Design review of the part shown in the three views and the two pictorial views. Dimensions are in mm from the part's minimum x, y and z. Give positions to 0.01 mm unless a question says otherwise; leave off trailing zeros. Loops run counter-clockwise (first coordinate to the right, second up) from the corner with the lowest first, then second, coordinate; pieces in that order, holes last.
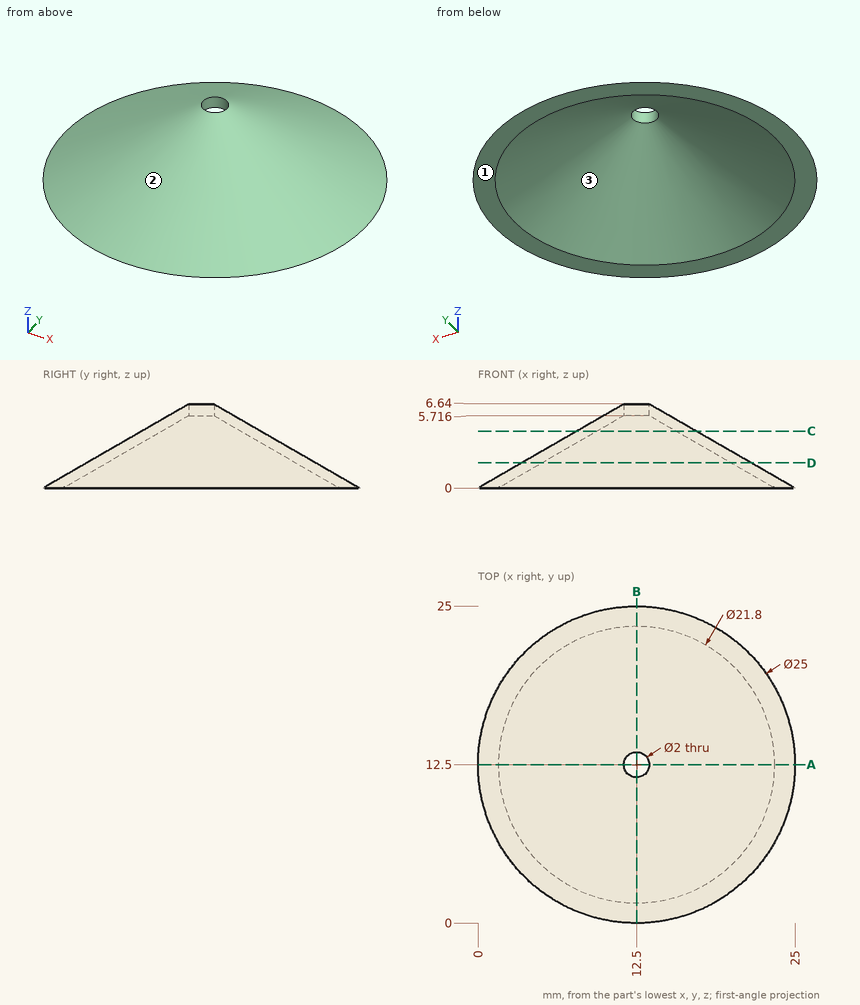
Q1. Insertion check: pin 1 (3 mm diameter, centred on x = 6, y = 15.5, fed in from +Z); pin 2 (1.6 mm diameter, centred on x = 12.5, y = 12.5, fed in from -Z); pin 3 (6 mm diameter, centred on x = 5, y = 19.5, fed in from +Z) (1 decimal); pin 4 (12 mm diameter, centred on x = 20.5, y = 8.5, fed in from +Z). Each pin has a flat end and moves straight along its axis. Give the tip position at first contact, or say it passes through.
Results:
pin 1: stops at z = 3.95
pin 2: passes through
pin 3: stops at z = 3
pin 4: stops at z = 5.52
Q2. Take a section at A-A (y = 12.5). Give the boundary of the cut face in (x, z) (1 decimal).
Results:
outline: (0, 0) - (1.6, 0) - (11.5, 5.7) - (11.5, 6.6) - close; (13.5, 5.7) - (23.4, 0) - (25, 0) - (13.5, 6.6) - close
Q3. Take a section at D-D (z = 2). Give the boundary of the cut face in (x, y) (1 decimal).
Results:
outline: circle Ø18.1 at (12.5, 12.5); hole circle Ø14.9 at (12.5, 12.5)
Q4. Take a section at C-C (z = 4.5). Give the boundary of the cut face in (x, y) (1 decimal).
Results:
outline: circle Ø9.4 at (12.5, 12.5); hole circle Ø6.2 at (12.5, 12.5)
Q5. Draft analysis for pull direction X (two halves, no side actions). For the marked faces 1, 2 and 3, state which applies: pulls with the +X half, pulls with the -X half, needs draft (parallel to the pull), parting line crosses it, or undercut.
Results:
face 1: needs draft
face 2: parting line crosses it
face 3: undercut
Q6. Wall thickness on line 1 (X direction, y = 7.5, z = 1.75) (1 decimal); line 2 (X direction, y = 18.75, z = 1) (1 decimal); line 3 (Y direction, x = 5.25, z = 0.5) (1 decimal): over which ranges is each line inside the solid? List them lowest first.
Results:
line 1: x = 4.5 to 6.4, 18.6 to 20.5
line 2: x = 3.7 to 5.8, 19.2 to 21.3
line 3: y = 3.4 to 5.6, 19.4 to 21.6
